Read the model definition and answer for the solid it produces. Units are mm, in the model's axes. A direction names the side the tool comes from. Coordinates: 2 decimals unless noted, no trailing zeros. Loops run counter-clockwise (first coordinate to the right, second up) from the corner with the lowest first, then second, coordinate; pieces in that order, holes last. Notation, with made-up numbers: (48, 17) -> (107, 17) arc R20 ccw to (107, 41) -> close; hole circle Ø3 at (59, 31). An arc over 180 degrees is marked (long way). Answer in a Markdown table with one row per item.
```python
from build123d import *

# Parameters (mm, degrees)
BOSS_EXTRUDE1_DEPTH        = 6.35
F_1_2_0_5_DIAMETER_HOLE1_D = 12.7


with BuildPart() as part:
    # Sketch1 → Boss-Extrude1 (new, symmetric)
    with BuildSketch(Plane.XY):
        Polygon((0, 38.14379681), (-88.9, 38.14379681), (-88.9, 190.54379681), (63.5, 190.54379681), (304.8, 101.6), (304.8, 0), (0, 0), align=None)
    extrude(amount=BOSS_EXTRUDE1_DEPTH, both=True)

    # 1/2 (0.5) Diameter Hole1 (through all)
    with Locations(Plane(origin=(-44.45, 139.74379681, 6.35), x_dir=(1, 0, 0), z_dir=(0, 0, 1))):
        with Locations((0, 0)):
            Hole(F_1_2_0_5_DIAMETER_HOLE1_D / 2)


solid = part.part
```
1. A cutting plane is placed at B-B on z = 0. Give the vertices of the cut face in (x, y), and give its area (3 significant figures).
A:
| item | result |
|---|---|
| outline | (-88.9, 38.14) -> (0, 38.14) -> (0, 0) -> (304.8, 0) -> (304.8, 101.6) -> (63.5, 190.54) -> (-88.9, 190.54) -> close; hole circle Ø12.7 at (-44.45, 139.74) |
| area | 60,800 mm2 |
2. Find the intervals of material crossed by probe 1 along Y at (x, z) = (-44.45, -2.5); probe 2 along X at (y, z) = (35, -5); probe 3 along Y at (x, z) = (-67, -4), in increasing order.
A:
| item | result |
|---|---|
| probe 1 | y = 38.14 to 133.39, 146.09 to 190.54 |
| probe 2 | x = 0 to 304.8 |
| probe 3 | y = 38.14 to 190.54 |
3. A cutting plane is placed at A-A on x = -44.45. Give the vertices of the cut face in (y, z), and give its area (3 significant figures).
A:
| item | result |
|---|---|
| outline | (38.14, -6.35) -> (133.39, -6.35) -> (133.39, 6.35) -> (38.14, 6.35) -> close; (146.09, -6.35) -> (190.54, -6.35) -> (190.54, 6.35) -> (146.09, 6.35) -> close |
| area | 1,770 mm2 |
4. The mould has two halves that part along X. Classify faces 3 (the flat face through (182.461, 146.695, 0.089)), 4 (the flat face through (155, 0, 0)), 5 (the flat face through (-88.9, 113, 0)), 6 (the cylindrical face through (-50.316, 137.312, -0.089)): pulls with the +X half, pulls with the -X half, needs draft (parallel to the pull), parting line crosses it, or undercut.
A:
| item | result |
|---|---|
| face 3 | pulls with the +X half |
| face 4 | needs draft |
| face 5 | pulls with the -X half |
| face 6 | undercut |
5. A cutting plane is placed at D-D on x = 256.5. Give the vertices of the cut face in (y, z).
A:
| item | result |
|---|---|
| outline | (0, -6.35) -> (119.4, -6.35) -> (119.4, 6.35) -> (0, 6.35) -> close |
6. A cutting plane is placed at C-C on y = 23. Give the vertices of the cut face in (x, z), and give its area (3 significant figures).
A:
| item | result |
|---|---|
| outline | (0, -6.35) -> (304.8, -6.35) -> (304.8, 6.35) -> (0, 6.35) -> close |
| area | 3,870 mm2 |
7. Given pin 1 Ø5 at (x, z) = (138, 4) entering from +Y; pin 2 Ø6 at (x, z) = (200.5, -1) entering from +Y; pin 3 Ø3 at (x, z) = (66.5, 2) entering from +Y, each flat-ended and moving along its own axis, determine where each tip first touches the part or whether it passes through.
A:
| item | result |
|---|---|
| pin 1 | stops at y = 164 |
| pin 2 | stops at y = 141.15 |
| pin 3 | stops at y = 189.99 |
8. A tool of negligible diameter and unlimited length cuts with its end or side. For faces 1 (the flat face through (-14, 190.544, 0)), 2 (the flat face through (-44, 38.144, 0)), from which of +Z, -Z, +X, -X, +Y, -Y can it reach the whole face along a straight path? Write none if from no direction.
A:
| item | result |
|---|---|
| face 1 | +Z, -Z, +X, -X, +Y |
| face 2 | +Z, -Z, -X, -Y |
